CAD build for the part. Positions are in the model's coordinates, mm. Face numbers are marked on the shaded views. A direction names the side the tool comes from. Round coordinates to 2 decimals unless told otherwise and drop trailing zeros. Loops run counter-clockwise (first coordinate to the right, second up) from the corner with the lowest first, then second, coordinate; pieces in that order, holes last. Notation, with made-up numbers: M 4,-36 L 17,-36 A25 cw 17,-17 Z; hole C 73.5,-20.75 d6. An arc over 180 degrees is marked long. Use one line per item in the form item = value.
from build123d import *

# Parameters (mm, degrees)
ESTRUSIONE_ESTRUSIONE1_DEPTH           = 100
RACCORDO1_R                            = 2
RACCORDO2_R                            = 4
FORO_SVASATO_PER_VITE_M4_1_D           = 4.5
FORO_SVASATO_PER_VITE_M4_1_DEPTH       = 188
FORO_SVASATO_PER_VITE_M4_1_CSINK_D     = 9.4
FORO_SVASATO_PER_VITE_M4_1_CSINK_ANGLE = 90
FORO_SVASATO_PER_VITE_M4_1_TIP         = 1.351936393


with BuildPart() as part:
    # Schizzo1 → Estrusione-Estrusione1 (new body)
    with BuildSketch(Plane.XY):
        Polygon((0, 0), (-2.5, 0), (-2.5, 11.5), (-8.5, 11.5), (-8.5, 35.5), (-6.5, 35.5), (-6.5, 13.5), (19, 13.5), (19, 10.5), (0, 10.5), align=None)
    extrude(amount=ESTRUSIONE_ESTRUSIONE1_DEPTH)

    # Raccordo1
    raccordo1_edges = [part.edges().sort_by_distance(p)[0] for p in [
        (-2.5, 11.5, 50),
        (-6.5, 13.5, 50),
    ]]
    fillet(raccordo1_edges, radius=RACCORDO1_R)

    # Raccordo2
    raccordo2_edges = [part.edges().sort_by_distance(p)[0] for p in [
        (-8.5, 11.5, 50),
    ]]
    fillet(raccordo2_edges, radius=RACCORDO2_R - 0.0001)  # a hair under: the kernel refuses the full size

    # Foro svasato per Vite M4-1
    with Locations(Plane.ZY.offset(2.5)):
        with Locations((85, 4.5), (15, 4.5)):
            CounterSinkHole(FORO_SVASATO_PER_VITE_M4_1_D / 2, FORO_SVASATO_PER_VITE_M4_1_CSINK_D / 2, depth=FORO_SVASATO_PER_VITE_M4_1_DEPTH, counter_sink_angle=FORO_SVASATO_PER_VITE_M4_1_CSINK_ANGLE)
            with Locations((0, 0, -(FORO_SVASATO_PER_VITE_M4_1_DEPTH + FORO_SVASATO_PER_VITE_M4_1_TIP / 2))):  # 118° drill point
                Cone(0, FORO_SVASATO_PER_VITE_M4_1_D / 2, FORO_SVASATO_PER_VITE_M4_1_TIP, mode=Mode.SUBTRACT)


solid = part.part
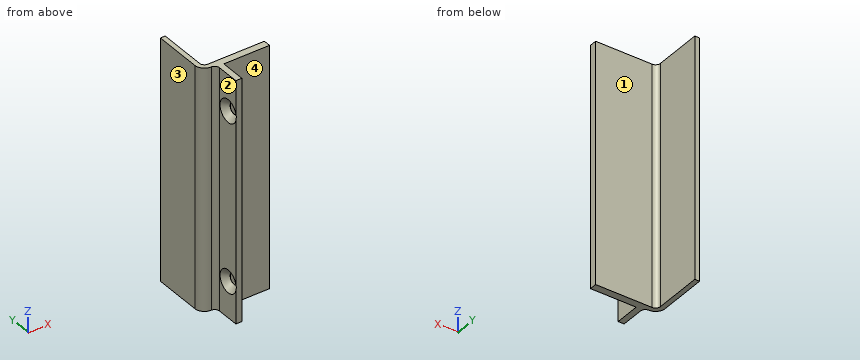
1. Tool access for the marked faces 1, 2, 3 and 4: list every direction of +Z, -Z, +X, -X, +Y, -Y with a clear straight run to the whole face (end or side of a thin tool).
Completed:
face_1 = +Z, -Z, +X, +Y
face_2 = +Z, -Z, -X, -Y
face_3 = +Z, -Z, -X, +Y, -Y
face_4 = +Z, -Z, +X, -Y
2. Cut at D-D on x = 8.25. Write the cut outline in (y, z).
Completed:
outline = M 10.5,0 L 13.5,0 L 13.5,100 L 10.5,100 Z
3. Probe line 1 along Y through (x, z) = (0.05, 85); line 2 along Z through (x, y) = (-1.5, 6); line 3 along X through (y, z) = (6, 69.5). List the from-to ranges inside material, lowest first. Write a range as from..to.
Completed:
line_1 = 10.5..13.5
line_2 = 0..11.62, 18.38..81.62, 88.38..100
line_3 = -2.5..0
4. Cut at B-B on y = 4.5. Write the cut outline in (x, z), and give its area (3 significant figures).
Completed:
outline = M -2.5,0 L 0,0 L 0,12.75 L -0.05,12.75 L -2.5,10.3 Z; M -2.5,19.7 L -0.05,17.25 L 0,17.25 L 0,82.75 L -0.05,82.75 L -2.5,80.3 Z; M -2.5,89.7 L -0.05,87.25 L 0,87.25 L 0,100 L -2.5,100 Z
area = 215 mm2
5. Drop flat-ended pins along their axis: P1, Ø8, axis at x = 15.5, z = 64, coming from the -Y side; P2, Ø6, axis at y = 4.5, z = 15, coming from the +X side; P3, Ø3, axis at x = 6.5, y = 8, coming from the +Z side; P4, Ø7.5, axis at y = 5, z = 62, coming from the -X side. Give the stop position or say it passes through.
Completed:
P1 = 10.5
P2 = 0
P3 = through
P4 = -2.5
